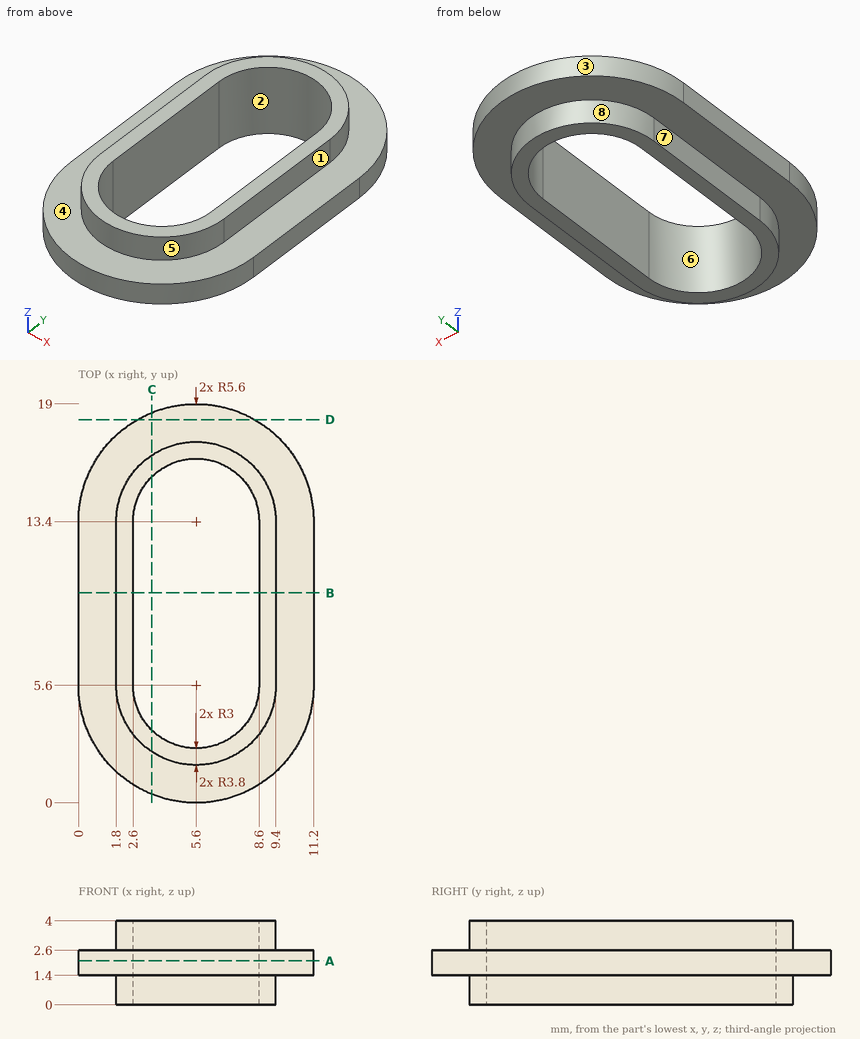
Part print with two shaded views. Sizes in mm from the minimum x, y, z corner. A direction names the side the tool comes from. Round coordinates to 2 decimals unless told otherwise and drop trailing zeros. Loops run counter-clockwise (first coordinate to the right, second up) from the corner with the lowest first, then second, coordinate; pieces in that order, holes last. Notation, with made-up numbers: M 39.5,26.25 L 59.5,26.25 A26 ccw 59.5,62.25 Z; hole C 7,46 d9. An arc over 180 degrees is marked long. Return JSON: item names as keys, results as strings. Group by question number.
(1) Drop flat-ended pins along their axis: P1, Ø1.1, axis at y = 8.5, z = 3.5, coming from the +X side; P2, Ø0.7, axis at y = 9.5, z = 3, coming from the -X side; P3, Ø1.5, axis at y = 14.5, z = 2, coming from the +X side. Give the stop position or say it passes through.
(2) Wall check: probe 1 along X at (y, z) = (8.25, 0.2); probe 2 along X at (y, z) = (13, 2.45); probe 3 along Z at (x, y) = (10.5, 14.5). Give the ranges that are in metal, low to high. Write a range as [from, to].
(3) Saw through at D-D, the plane y = 18.25. List the corners of the cut face in (x, z), and give its area (3 significant figures).
(4) Saw through at C-C, the plane x = 3.5. List the corners of the cut face in (y, z).
(5) Saw through at B-B, the plane y = 10. List the corners of the cut face in (x, z), and give its area (3 significant figures).
(6) Saw through at A-A, the plane z = 2.1. List the corners of the cut face in (x, y).
(7) Tool access for the marked faces 4, 5, 6, 7 and 8: list every direction of +Z, -Z, +X, -X, +Y, -Y with a clear straight run to the whole face (end or side of a thin tool).
(8) Mould opens along Y. For the marked faces 1, 2 and 3 say: +Y half, -Y half, draft (parallel to the pull), parting line (faces both ways), or undercut.
Answer list:
{
 "1": {"P1": "x = 9.4", "P2": "x = 1.8", "P3": "x = 11.19"},
 "2": {"probe 1": "[1.8, 2.6], [8.6, 9.4]", "probe 2": "[0, 2.6], [8.6, 11.2]", "probe 3": "[1.4, 2.6]"},
 "3": {"outline": "M 2.8,1.4 L 8.4,1.4 L 8.4,2.6 L 2.8,2.6 Z", "area": "6.72 mm2"},
 "4": {"outline": "M 0.41,1.4 L 2.43,1.4 L 2.43,0 L 3.46,0 L 3.46,4 L 2.43,4 L 2.43,2.6 L 0.41,2.6 Z; M 15.54,0 L 16.57,0 L 16.57,1.4 L 18.59,1.4 L 18.59,2.6 L 16.57,2.6 L 16.57,4 L 15.54,4 Z"},
 "5": {"outline": "M 0,1.4 L 1.8,1.4 L 1.8,0 L 2.6,0 L 2.6,4 L 1.8,4 L 1.8,2.6 L 0,2.6 Z; M 8.6,0 L 9.4,0 L 9.4,1.4 L 11.2,1.4 L 11.2,2.6 L 9.4,2.6 L 9.4,4 L 8.6,4 Z", "area": "10.7 mm2"},
 "6": {"outline": "M 0,5.6 A5.6 ccw 11.2,5.6 L 11.2,13.4 A5.6 ccw 0,13.4 Z; hole M 2.6,5.6 A3 ccw 8.6,5.6 L 8.6,13.4 A3 ccw 2.6,13.4 Z"},
 "7": {"face 4": "+Z", "face 5": "+Z, -Y", "face 6": "+Z, -Z", "face 7": "-Z, -X, +Y, -Y", "face 8": "-Z, +Y"},
 "8": {"face 1": "draft", "face 2": "undercut", "face 3": "+Y half"}
}
